Verification items for the finished model (mm, model axes). A direction names the side the tool comes from. Coordinates: 2 decimals unless noted, no trailing zeros. Loops run counter-clockwise (first coordinate to the right, second up) from the corner with the lowest first, then second, coordinate; pieces in that order, holes last. Notation, with made-up numbers: (64.25, 58) - (70.25, 58) arc R14 cw to (70.25, 72) - close; hole circle Ø4 at (3, 38.25). An arc over 180 degrees is marked (long way). One line per item, written item: value. Start each with the question number.
(1) Draft check along X on faces 4 (the face through (20, 1, -1)), 5 (the face through (-10.66, 1.01, 16.46)), 6 (the face through (-0.148, 0.986, -22.125)). Enter one of: +X half, -X half, draft (parallel to the pull), parting line (faces both ways), or undercut.
(2) Thickness scan on probe 1 along X at (y, z) = (1.65, -17.5); probe 2 along X at (y, z) = (1.9, -14.5); probe 3 along Z at (x, y) = (-10, 1.35). Record the ranges inside material, lowest first. Write a range as [from, to].
(3) Gauge pin test, flat ends, axial feed: P1, Ø3, axis at x = -14.5, z = -8.5, coming from the -Y side; P2, Ø0.6, axis at x = -19, y = 1, coming from the +Z side. Record the tip position at first contact, or that the pin passes through.
(4) Section check D-D (x = 16). Record the boundary of the cut face in (y, z), plus the area to 3 significant figures.
(5) Section check A-A (z = 10.5). Record the boundary of the cut face in (x, y).
(6) Set-up check for faces 1 (the face through (-8.575, 1.014, -14.824)), 2 (the face through (-19.234, 0.986, -10.934)), 3 (the face through (-20, 1, 1)): record each of +Z, -Z, +X, -X, +Y, -Y from which the full face is reachable in a straight line by a thin tool's end or side.
(7) Section check C-C (z = 16). Record the boundary of the cut face in (x, y), plus the area to 3 significant figures.
(8) Section check B-B (x = -18). Record the boundary of the cut face in (y, z), plus the area to 3 significant figures.
Autodesk Inventor part; units mm, degrees
ref_plane "YZ Plane" through (0, 0, 0) normal (1, 0, 0) x (0, 1, 0)
ref_plane "XZ Plane" through (0, 0, 0) normal (0, 1, 0) x (-1, 0, 0)
ref_plane "XY Plane" through (0, 0, 0) normal (0, 0, 1) x (1, 0, 0)
sketch "Sketch1" plane through (0, 0, 0) normal (0, 1, 0) x (-1, 0, 0)
  circle A0 centre (0, 0) radius 22.125
  circle A1 centre (0, 0) radius 12.125
  dimension "d0" = 44.25
  dimension "d1" = 24.25
extrude "Extrusion1" add sketch "Sketch1" along normal blind 2
sketch "Sketch2" plane through (0, 2, 0) normal (0, 1, 0) x (1, 0, 0)
  line L0 (-27.125, -1) -> (-17.125, -1)
  line L1 (-17.125, -1) -> (-17.125, 1)
  line L2 (-17.125, 1) -> (-27.125, 1)
  line L3 (-27.125, 1) -> (-27.125, -1)
  point P0 (0, 0)
  dimension "d4" = 1
  dimension "d5" = 2
  dimension "d6" = 10
  dimension "d7" = 17.125
extrude "Extrusion2" cut sketch "Sketch2" against normal blind 2
pattern_circular "Circular Pattern1" count 6 over 360 about axis through (0, -10, 0) along (0, 1, 0) of "Extrusion2"
sketch "Sketch3" plane through (0, 2, 0) normal (0, 1, 0) x (1, 0, 0)
  circle A0 centre (-6.9282, -4) radius 5.5
  line L0 (-6.9282, -4) -> (0, 0) construction
  line L1 (-37.5572, 0) -> (32.0456, 0)
  dimension "d13" = 11
  dimension "d14" = 30
  dimension "d15" = 4
extrude "Extrusion3" cut sketch "Sketch3" against normal blind 2
pattern_circular "Circular Pattern2" count 6 over 360 about axis through (0, -10, 0) along (0, 1, 0) of "Extrusion3"
properties part number "Ring_n4"
Responses:
1. face 4: draft
1. face 5: undercut
1. face 6: parting line
2. probe 1: x = [-13.54, -11.26], [-8.95, 8.95], [11.26, 13.54]
2. probe 2: x = [-16.71, -9.53], [-9.14, 9.14], [9.53, 16.71]
2. probe 3: z = [-19.74, -19.32], [-15.32, -8.56], [8.56, 15.32], [19.32, 19.74]
3. P1: stops at y = 0
3. P2: stops at z = 11.82
4. outline: (0, -15.28) - (2, -15.28) - (2, 15.28) - (0, 15.28) - close
4. area: 61.1 mm²
5. outline: (-19.47, 0) - (-6.06, 0) - (-6.06, 2) - (-19.47, 2) - close; (6.06, 0) - (19.47, 0) - (19.47, 2) - (6.06, 2) - close
6. face 1: +Y, -Y
6. face 2: -Z, -X, +Y, -Y
6. face 3: -X, +Y, -Y
7. outline: (-15.28, 0) - (-10.39, 0) - (-10.39, 2) - (-15.28, 2) - close; (-8.08, 0) - (8.08, 0) - (8.08, 2) - (-8.08, 2) - close; (10.39, 0) - (15.28, 0) - (15.28, 2) - (10.39, 2) - close
7. area: 51.9 mm²
8. outline: (0, -12.87) - (2, -12.87) - (2, -1) - (0, -1) - close; (0, 1) - (2, 1) - (2, 12.87) - (0, 12.87) - close
8. area: 47.5 mm²
